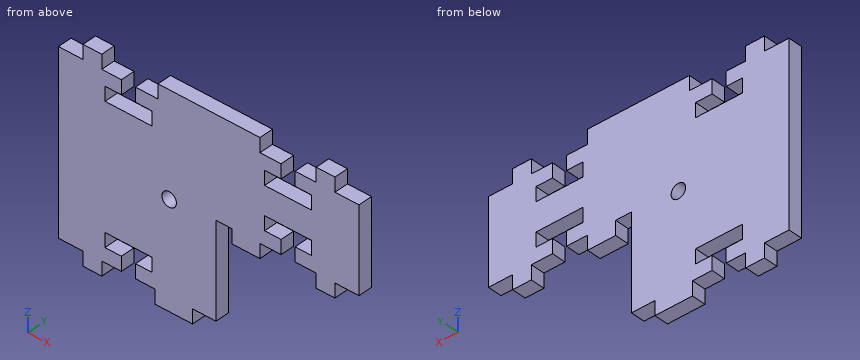
from build123d import *

# Parameters (mm, degrees)
SKETCH1_R           = 1.55
BOSS_EXTRUDE1_DEPTH = 3


with BuildPart() as part:
    # Sketch1 → Boss-Extrude1 (new body)
    with BuildSketch(Plane(origin=(0, 0, 0), x_dir=(1, 0, 0), z_dir=(0, 1, 0))):
        Polygon((74.683753319, 219.09410576), (69.551868319, 219.09410576), (69.551868319, 216.09410576), (65.551868319, 216.09410576), (65.551868319, 219.09410576), (61.051868319, 219.09410576), (61.051868319, 222.09410576), (64.551868319, 222.09410576), (64.551868319, 225.09410576), (54.551868319, 225.09410576), (54.551868319, 222.09410576), (58.051868319, 222.09410576), (58.051868319, 219.09410576), (53.551868319, 219.09410576), (53.551868319, 216.09410576), (31.815637319, 216.09410576), (31.815637319, 219.09410576), (26.999695069, 219.09410576), (26.999695069, 222.09410576), (30.499695069, 222.09410576), (30.499695069, 225.09410576), (20.499695069, 225.09410576), (20.499695069, 222.09410576), (23.999695069, 222.09410576), (23.999695069, 219.09410576), (19.815637319, 219.09410576), (19.815637319, 216.09410576), (15.815637319, 216.09410576), (15.815637319, 219.09410576), (10.583753319, 219.09410576), (10.583753319, 257.09410576), (15.815637319, 257.09410576), (15.815637319, 260.09410576), (19.815637319, 260.09410576), (19.815637319, 257.09410576), (23.999695069, 257.09410576), (23.999695069, 254.09410576), (20.499695069, 254.09410576), (20.499695069, 251.09410576), (30.499695069, 251.09410576), (30.499695069, 254.09410576), (26.999695069, 254.09410576), (26.999695069, 257.09410576), (31.183752819, 257.09410576), (31.183752819, 260.09410576), (39.183752819, 260.09410576), (39.183752819, 257.09410576), (44.183752819, 257.09410576), (44.183752819, 237.09410576), (47.551868319, 237.09410576), (47.551868319, 240.09410576), (53.551868319, 240.09410576), (53.551868319, 237.09410576), (58.051868319, 237.09410576), (58.051868319, 234.09410576), (54.551868319, 234.09410576), (54.551868319, 231.09410576), (64.551868319, 231.09410576), (64.551868319, 234.09410576), (61.051868319, 234.09410576), (61.051868319, 237.09410576), (65.551868319, 237.09410576), (65.551868319, 240.09410576), (69.551868319, 240.09410576), (69.551868319, 237.09410576), (74.683753319, 237.09410576), align=None)
        with Locations(Location((34.183752819, 237.84410576, 0), (0, 0, 270))):
            Circle(SKETCH1_R, mode=Mode.SUBTRACT)
    extrude(amount=BOSS_EXTRUDE1_DEPTH)


solid = part.part
The model under review builds one solid part; all positions refer to its coordinate system, in mm. Give positions to 0.01 mm unless a question says otherwise; leave off trailing zeros. Write each loop counter-clockwise with the first axis right and the second up, starting at its lowest first coordinate (ties: lowest second). Pieces come first, ordered by that corner, then holes. Notation, with made-up numbers: M -39.75,-10.75 L -12.75,-10.75 A8 ccw -12.75,-5.75 Z; hole C 45.25,54.5 d10. An arc over 180 degrees is marked long. One line per question, with ' | ' between items. Start each with the question number.
Item 1: We need section B-B on z = -232.5. Write out the cut boundary in (x, y), plus the area to 3 significant figures.
Item 2: Wall thickness on line 1 (X direction, y = 2.4, z = -220); line 2 (X direction, y = 1.2, z = -218.5); line 3 (X direction, y = 1.95, z = -253.5): over which ranges is each line inside the solid? List them lowest first. Write a range as from..to.
Item 3: We need section D-D on z = -242. Write out the cut boundary in (x, y).
Item 4: We need section A-A on x = 21.5. Write out the cut boundary in (y, z).
Item 5: For pin 1 (0.9 mm diameter, centred on x = 22, y = 1.5, fed in from +Z); pin 2 (0.9 mm diameter, centred on x = 28.5, y = 2, fed in from -Z); pin 3 (0.9 mm diameter, centred on x = 67, y = 1, fed in from -Z), all flat-tipped, find the tip position at first contact; note any pin that passes through.
Item 6: We need section C-C on z = -252. Write out the cut boundary in (x, y).
Results found:
1) outline: M 10.58,0 L 54.55,0 L 54.55,3 L 10.58,3 Z; M 64.55,0 L 74.68,0 L 74.68,3 L 64.55,3 Z | area: 162 mm2
2) line 1: x = 10.58..24, 27..58.05, 61.05..74.68 | line 2: x = 15.82..19.82, 31.82..53.55, 65.55..69.55 | line 3: x = 10.58..20.5, 30.5..44.18
3) outline: M 10.58,0 L 44.18,0 L 44.18,3 L 10.58,3 Z
4) outline: M 0,-257.09 L 3,-257.09 L 3,-254.09 L 0,-254.09 Z; M 0,-251.09 L 3,-251.09 L 3,-225.09 L 0,-225.09 Z; M 0,-222.09 L 3,-222.09 L 3,-219.09 L 0,-219.09 Z
5) pin 1: stops at z = -219.09 | pin 2: stops at z = -257.09 | pin 3: stops at z = -240.09
6) outline: M 10.58,0 L 20.5,0 L 20.5,3 L 10.58,3 Z; M 30.5,0 L 44.18,0 L 44.18,3 L 30.5,3 Z
